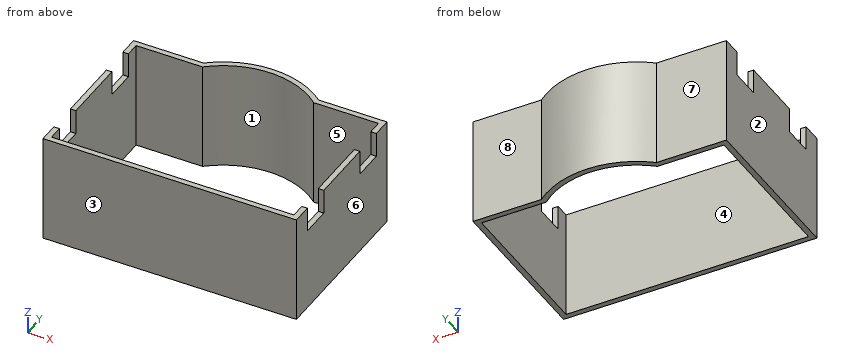
from build123d import *

# Parameters (mm, degrees)
BOSS_EXTRUDE2_DEPTH = 49.8602
SHELL2_T            = 2.54
SKETCH4_W           = 2.54
SKETCH4_H           = 14.004037607
SKETCH4_H_2         = 14.000022482
SKETCH4_H_3         = 14.004058035
CUT_EXTRUDE1_DEPTH  = 11.43


with BuildPart() as part:
    # Sketch2 → Boss-Extrude2 (new body)
    with BuildSketch(Plane.XY):
        with BuildLine():
            Line((20.510960331, 69.60596379), (50.371443222, 69.60596379))
            Line((50.371443222, 69.60596379), (50.371443222, -1.977240525))
            Line((50.371443222, -1.977240525), (-61.38356009, -1.977240525))
            Line((-61.38356009, -1.977240525), (-61.38356009, 69.60596379))
            Line((-61.38356009, 69.60596379), (-30.761077997, 69.60596379))
            ThreePointArc((-30.761077997, 69.60596379), (-5.125058833, 79.163961442), (20.510960331, 69.60596379))
        make_face()
    extrude(amount=BOSS_EXTRUDE2_DEPTH)

    # Shell2
    shell2_openings = [part.faces().sort_by_distance(p)[0] for p in [
        (-5.490717903, 35.411141446, 0),
        (-5.490717903, 35.411141446, 49.8602),
    ]]
    offset(amount=SHELL2_T, openings=shell2_openings, kind=Kind.INTERSECTION)

    # Sketch4 → Cut-Extrude1 (cut)
    with BuildSketch(Plane.XY.offset(49.8602)):
        with Locations((-62.65356009, 56.116943469)):
            Rectangle(SKETCH4_W, SKETCH4_H)
        with Locations((-62.65356009, 11.668972532)):
            Rectangle(SKETCH4_W, SKETCH4_H_2)
        with Locations((51.641443222, 56.116953683)):
            Rectangle(SKETCH4_W, SKETCH4_H_3)
        with Locations((51.641443222, 11.668972532)):
            Rectangle(SKETCH4_W, SKETCH4_H_2)
    extrude(amount=-CUT_EXTRUDE1_DEPTH, mode=Mode.SUBTRACT)


solid = part.part
Could you check a few things on this model? Use its own coordinates, in mm. Face numbers are marked on the shaded views. A direction names the side the tool comes from. Give positions to 0.01 mm unless a question says otherwise; leave off trailing zeros. Loops run counter-clockwise (first coordinate to the right, second up) from the corner with the lowest first, then second, coordinate; pieces in that order, holes last. Notation, with made-up numbers: M 23.5,21.5 L 61.5,21.5 A17 ccw 61.5,54.5 Z; hole C 75,66.25 d7. An arc over 180 degrees is marked long. Answer as a JSON object with one key per item and string values.
Q1. Suppose I cut it at C-C, the plane x = -39. List the corners of the cut face in (y, z) for me, plus the area to 3 significant figures.
Values found:
{"outline": "M -4.52,0 L -1.98,0 L -1.98,49.86 L -4.52,49.86 Z; M 69.61,0 L 72.15,0 L 72.15,49.86 L 69.61,49.86 Z", "area": "253 mm²"}
Q2. If we mould it in two halves opening along X, with no side actions, what happens to the marked faces 1, 2, 3 and 4? For each: pulls with the +X half, pulls with the -X half, needs draft (parallel to the pull), parting line crosses it, or undercut.
Values found:
{"face 1": "undercut", "face 2": "pulls with the -X half", "face 3": "needs draft", "face 4": "undercut"}
Q3. For P1, Ø1.3, axis at x = 51.5, y = 54.5, coming from the +Z side; P2, Ø3, axis at x = 52, z = 41.5, coming from the +Y side, each with a flat end and sliding along its axis, tell me the tip position at first contact or that it passes through.
Values found:
{"P1": "stops at z = 38.43", "P2": "stops at y = 72.15"}
Q4. Suppose I cut it at A-A, the plane y = 25.5. List the corners of the cut face in (x, z) for me.
Values found:
{"outline": "M -63.92,0 L -61.38,0 L -61.38,49.86 L -63.92,49.86 Z; M 50.37,0 L 52.91,0 L 52.91,49.86 L 50.37,49.86 Z"}
Q5. Suppose I cut it at D-D, the plane z = 20. List the corners of the cut face in (x, y) for me, plus the area to 3 significant figures.
Values found:
{"outline": "M -63.92,-4.52 L 52.91,-4.52 L 52.91,72.15 L 21.44,72.15 A41.7 ccw -31.69,72.15 L -63.92,72.15 Z; hole M -61.38,-1.98 L 50.37,-1.98 L 50.37,69.61 L 20.51,69.61 A39.16 ccw -30.76,69.61 L -61.38,69.61 Z", "area": "969 mm²"}
Q6. Suppose I cut it at B-B, the plane z = 42. List the corners of the cut face in (x, y) for me, plus the area to 3 significant figures.
Values found:
{"outline": "M -63.92,-4.52 L 52.91,-4.52 L 52.91,4.67 L 50.37,4.67 L 50.37,-1.98 L -61.38,-1.98 L -61.38,4.67 L -63.92,4.67 Z; M -63.92,18.67 L -61.38,18.67 L -61.38,49.11 L -63.92,49.11 Z; M -63.92,63.12 L -61.38,63.12 L -61.38,69.61 L -30.76,69.61 A39.16 cw 20.51,69.61 L 50.37,69.61 L 50.37,63.12 L 52.91,63.12 L 52.91,72.15 L 21.44,72.15 A41.7 ccw -31.69,72.15 L -63.92,72.15 Z; M 50.37,18.67 L 52.91,18.67 L 52.91,49.11 L 50.37,49.11 Z", "area": "826 mm²"}
Q7. If I drill on probe 1 along X at (y, z) = (33, 45); probe 2 along Y at (x, z) = (-49, 9); probe 3 along Y at (x, z) = (-4.5, 15), over which ranges is the centre line in solid material (lowest first)? Write a range as [from, to].
Values found:
{"probe 1": "x = [-63.92, -61.38], [50.37, 52.91]", "probe 2": "y = [-4.52, -1.98], [69.61, 72.15]", "probe 3": "y = [-4.52, -1.98], [79.16, 81.7]"}
Q8. For the marked faces 5, 6, 7 and 8, which set-ups out of +Z, -Z, +X, -X, +Y, -Y let a thin tool reach every point of the face, with its end or its side?
Values found:
{"face 5": "+Z, -Z", "face 6": "+Z, -Z, +X, +Y, -Y", "face 7": "+Z, -Z, -X, +Y", "face 8": "+Z, -Z, +X, +Y"}
